from build123d import *

# Parameters (mm, degrees)
SKETCH_1_R               = 31.25
SKETCH_1_R_2             = 4
EXTRUDE_1_DEPTH          = 6
SKETCH_2_R               = 10
SKETCH_2_R_2             = 4
EXTRUDE_2_DEPTH          = 10
SKETCH_3_R               = 1
CUT_EXTRUDE_1_DEPTH      = 32.25
CUT_EXTRUDE_1_DEPTH_BACK = 32.25
SKETCH_4_R               = 1
CUT_EXTRUDE_2_DEPTH      = 32.25
CUT_EXTRUDE_2_DEPTH_BACK = 32.25


with BuildPart() as part:
    # Эскиз1 → Бобышка-Вытянуть1 (new body)
    with BuildSketch(Plane.XY):
        Circle(SKETCH_1_R)
        Circle(SKETCH_1_R_2, mode=Mode.SUBTRACT)
    extrude(amount=EXTRUDE_1_DEPTH)

    # Эскиз2 → Бобышка-Вытянуть2 (add)
    with BuildSketch(Plane.XY.offset(6)):
        Circle(SKETCH_2_R)
        Circle(SKETCH_2_R_2, mode=Mode.SUBTRACT)
    extrude(amount=EXTRUDE_2_DEPTH)

    # Эскиз3 → Вырез-Вытянуть1 (cut, two sides)
    with BuildSketch(Plane(origin=(0, 0, 0), x_dir=(1, 0, 0), z_dir=(0, 1, 0))) as cut_extrude_1_sk:
        with Locations((0, -9)):
            Circle(SKETCH_3_R)
    extrude(amount=CUT_EXTRUDE_1_DEPTH, mode=Mode.SUBTRACT)
    extrude(cut_extrude_1_sk.sketch, amount=-CUT_EXTRUDE_1_DEPTH_BACK, mode=Mode.SUBTRACT)

    # Эскиз4 → Вырез-Вытянуть2 (cut, two sides)
    with BuildSketch(Plane(origin=(0, 0, 0), x_dir=(0, 0, -1), z_dir=(1, 0, 0))) as cut_extrude_2_sk:
        with Locations((-13, 0)):
            Circle(SKETCH_4_R)
    extrude(amount=CUT_EXTRUDE_2_DEPTH, mode=Mode.SUBTRACT)
    extrude(cut_extrude_2_sk.sketch, amount=-CUT_EXTRUDE_2_DEPTH_BACK, mode=Mode.SUBTRACT)


solid = part.part
Can you work these out from the model? Positions are in its coordinate system, mm. A direction names the side the tool comes from. Round coordinates to 2 decimals unless told otherwise and drop trailing zeros. Loops run counter-clockwise (first coordinate to the right, second up) from the corner with the lowest first, then second, coordinate; pieces in that order, holes last. Notation, with made-up numbers: (-15, 26) - (12, 26) arc R12 ccw to (12, 31) - close; hole circle Ø11 at (-37.75, -0.5). An arc over 180 degrees is marked (long way). Answer in a Markdown table with one row per item. Add a question column.
Q1. I need wall thicknesses on L1, parallel to Z at x = 0, y = -7; L2, parallel to Y at x = 0, z = 11.25; L3, parallel to Z at x = -11, y = 20.5. Which ranges of each line are inside material? Lowest first, please.
Q2. We'd pull the mould along Y, two halves only. Please class faces 1 (the cylindrical face through (-31.22, 1.37, 2.96)), 2 (the cylindrical face through (7, 0, 12)), 3 (the flat face through (-7.4, 7.4, 6)): pulls with the +Y half, pulls with the -Y half, needs draft (parallel to the pull), parting line crosses it, or undercut.
Q3. I want a section at D-D on y = 6.5. List the corners of the cut face in (x, z) for me.
Q4. Which directions (+Z, -Z, +X, -X, +Y, -Y) give clear straight access to the entire face, cutting with the end or side of a thin tool? Please do faces 4 (the cylindrical face through (9.237, -3.83, 10.93)), 5 (the cylindrical face through (0, 7, 8)).
Q5. I want a section at B-B on y = 0. List the corners of the cut face in (x, z) for me, and give its area (3 significant figures).
Q6. I want a section at A-A on x = 0. List the corners of the cut face in (y, z) for me.
Q7. For pin 1 Ø3 at (y, z) = (9.5, 14.5) entering from -X; pin 2 Ø6.5 at (x, y) = (0, 0) entering from +Z; pin 3 Ø8 at (y, z) = (-23, 5) entering from +X; pin 4 Ø3 at (y, z) = (0, 13) entering from +X, each with a flat end and sliding along its axis, tell me the tip position at first contact or that it passes through.
Q8. I want a section at C-C on z = 9. List the corners of the cut face in (x, y) for me, and give its area (3 significant figures).
A:
| question | item | result |
|---|---|---|
| 1 | L1 | 0 to 8, 10 to 16 |
| 1 | L2 | -10 to -4, 4 to 10 |
| 1 | L3 | 0 to 6 |
| 2 | face 1 | parting line crosses it |
| 2 | face 2 | undercut |
| 2 | face 3 | needs draft |
| 3 | outline | (-30.57, 0) - (30.57, 0) - (30.57, 6) - (7.6, 6) - (7.6, 16) - (-7.6, 16) - (-7.6, 6) - (-30.57, 6) - close; hole circle Ø2 at (0, 9) |
| 4 | face 4 | +Z |
| 4 | face 5 | +Y, -Y |
| 5 | outline | (-31.25, 0) - (-4, 0) - (-4, 12) - (-10, 12) - (-10, 6) - (-31.25, 6) - close; (-10, 14) - (-4, 14) - (-4, 16) - (-10, 16) - close; (4, 0) - (31.25, 0) - (31.25, 6) - (10, 6) - (10, 12) - (4, 12) - close; (4, 14) - (10, 14) - (10, 16) - (4, 16) - close |
| 5 | area | 423 mm^2 |
| 6 | outline | (-31.25, 0) - (-4, 0) - (-4, 8) - (-10, 8) - (-10, 6) - (-31.25, 6) - close; (-10, 10) - (-4, 10) - (-4, 16) - (-10, 16) - close; (4, 0) - (31.25, 0) - (31.25, 6) - (10, 6) - (10, 8) - (4, 8) - close; (4, 10) - (10, 10) - (10, 16) - (4, 16) - close |
| 7 | pin 1 | x = -6 |
| 7 | pin 2 | through |
| 7 | pin 3 | x = 24.81 |
| 7 | pin 4 | x = 10 |
| 8 | outline | (-1, -9.95) - (-1, -3.87) arc R4 cw to (-1, 3.87) - (-1, 9.95) arc R10 ccw to start; (1, -9.95) arc R10 ccw to (1, 9.95) - (1, 3.87) arc R4 cw to (1, -3.87) - close |
| 8 | area | 240 mm^2 |
